Read the model definition and answer for the solid it produces. Units are mm, in the model's axes. Give positions to 0.01 mm unless a question says otherwise; leave off trailing zeros. Write each loop counter-clockwise with the first axis right and the second up, starting at its lowest first coordinate (ties: lowest second). Pieces come first, ordered by that corner, then holes. Notation, with made-up numbers: M -19,-8 L 17,-8 A11 cw 17,12 Z; hole C -18.75,79 d10. An arc over 180 degrees is marked long. Use a Markdown table: item, result. Add a question column.
Item 1: Given P1, Ø0.5, axis at y = -0.5, z = 165.5, coming from the -X side, flat-ended and moving along its own axis, determine where the tip first touches the part or whether it passes through.
Item 2: A cutting plane is placed at A-A on z = 153.5. Determine the outline of the cut face in (x, y).
Item 3: A cutting plane is placed at B-B on z = 75.5. Determine the outline of the cut face in (x, y), then the cut area to 3 significant figures.
Item 4: Consider probe 1 along Z at (x, y) = (22, -0.55); probe 2 along Z at (x, y) = (15, -0.3); probe 3 along X at (y, z) = (-1.1, 206). Determine where each line is inside the solid, lowest interval first. Write a range as [from, to].
from build123d import *

# Parameters (mm, degrees)
F0_W     = 10.2457383797
F0_H     = 20.3
F0_W_2   = 2.4
F0_H_2   = 7.2
F0_H_3   = 11.2
F1_DEPTH = 1.6
F2_SIZE  = 0.5
F3_R     = 0.94999


# Not quite as in the source:
# - a fillet or chamfer is up to 0.001 mm smaller than in the source, because OpenCascade refuses the exact size


with BuildPart() as f1:
    # F0 (on Front) → F1 (new body)
    with BuildSketch(Plane.XZ):
        Polygon((0, 79.96), (0, 0), (167, 0), (167, 4), (164, 4), (164, 98), (167, 98), (167, 102), (160, 102), (160, 132), (167, 132), (167, 136), (164, 136), (164, 144), (167, 144), (167, 147.96), (166, 147.96), (166, 202.96), (167, 202.96), (167, 206.96), (164, 206.96), (164, 229.96), (167, 229.96), (167, 233.96), (0, 233.96), (0, 229.96), (10, 229.96), (10, 196.0979268551), (23.6, 196.0979268551), (23.6, 188.0729268551), (33.8457383797, 188.0729268551), (33.8457383797, 167.7729268551), (23.6, 167.7729268551), (23.6, 160.0979268551), (10, 160.0979268551), (10, 79.96), align=None)
        with Locations((28.7228691898, 177.9229268551)):
            Rectangle(F0_W, F0_H)
        Polygon((10, 174.9729268551), (10, 167.7729268551), (23.6, 167.7729268551), (23.6, 188.0729268551), (10, 188.0729268551), (10, 176.8729268551), (16, 176.8729268551), (16, 174.9729268551), align=None)
        with Locations((8.8, 171.3729268551)):
            Rectangle(F0_W_2, F0_H_2)
        with Locations((8.8, 182.4729268551)):
            Rectangle(F0_W_2, F0_H_3)
    extrude(amount=F1_DEPTH)

    # F2
    f2_edges = [f1.edges().sort_by_distance(p)[0] for p in [
        (7.6, -0.8, 167.772927),
        (7.6, -0.8, 174.972927),
        (7.6, -0.8, 176.872927),
        (7.6, -0.8, 188.072927),
    ]]
    chamfer(f2_edges, length=F2_SIZE)

    # F3 (radius 0.95 in the source; OpenCascade refuses exactly that, so slightly less here)
    f3_edges = [f1.edges().sort_by_distance(p)[0] for p in [
        (16, -0.8, 176.872927),
        (16, -0.8, 174.972927),
    ]]
    fillet(f3_edges, radius=F3_R)


solid = f1.part
Filled in:
| question | item | result |
|---|---|---|
| 1 | P1 | x = 23.6 |
| 2 | outline | M 10,-1.6 L 166,-1.6 L 166,0 L 10,0 Z |
| 3 | outline | M 0,-1.6 L 164,-1.6 L 164,0 L 0,0 Z |
| 3 | area | 262 mm² |
| 4 | probe 1 | [0, 160.1], [167.77, 188.07], [196.1, 233.96] |
| 4 | probe 2 | [0, 160.1], [167.77, 174.97], [176.87, 188.07], [196.1, 233.96] |
| 4 | probe 3 | [10, 167] |
